Here's how the part is built. I have some questions about the finished solid (model axes, mm). Face numbers are marked on the shaded views. A direction names the side the tool comes from. Coordinates: 2 decimals unless noted, no trailing zeros. Loops run counter-clockwise (first coordinate to the right, second up) from the corner with the lowest first, then second, coordinate; pieces in that order, holes last.
Autodesk Fusion 360 part; units mm, degrees
sketch "Sketch1" plane through (0, 0, 0) normal (0, 0, 1) x (1, 0, 0)
  circle A0 centre (0, 0) radius 50
  circle A1 centre (0, 0) radius 67.5
  line L0 (-188.7298, 10) -> (-172.9129, 10)
  line L1 (-188.7147, -10.0585) -> (-172.8873, -10.0585)
  arc A2 (-172.8873, -10.0585) -> (-172.9129, 10) centre (-150, 0) ccw
  line L2 (190, -0.0314) -> (190, 0.0314)
  line L3 (188.7379, 9.9686) -> (172.9266, 9.9686)
  line L4 (188.7216, -10.0319) -> (172.8989, -10.0319)
  arc A3 (190, -0.0314) -> (190, 0.0314) centre (150, 0) ccw
  arc A4 (172.9266, 9.9686) -> (172.8989, -10.0319) centre (150, 0) ccw
  spline S0 degree 5 poles (-140.0807, 38.7506) (-138.5307, 38.3538) (-135.4703, 37.4053) (-128.0478, 36.7264) (-108.2202, 39.6197) (-74.7434, 48.8035) (-51.6098, 57.8401) (-40.0528, 63.8063) (-33.7446, 67.0737) (-30.5053, 68.5159) knots 0 0 0 0 0 0 0.2 0.4 0.6 0.8 1 1 1 1 1 1
  line L5 (-43.0547, 62.9285) -> (-17.9559, 74.1033)
  spline S1 degree 5 poles (-140.0807, -38.7506) (-138.5307, -38.3538) (-135.4703, -37.4053) (-127.9422, -36.808) (-107.6532, -40.0429) (-73.5767, -49.609) (-50.5343, -58.4957) (-39.5693, -64.0411) (-33.8156, -67.0222) (-30.867, -68.3537) knots 0 0 0 0 0 0 0.2 0.4 0.6 0.8 1 1 1 1 1 1
  line L6 (-42.1759, -63.2468) -> (-19.558, -73.4606)
  arc A5 (-188.7147, -10.0585) -> (-140.0807, -38.7506) centre (-150, 0) ccw
  arc A6 (-140.0807, 38.7506) -> (-188.7298, 10) centre (-150, 0) ccw
  spline S2 degree 5 poles (140.0807, 38.7506) (138.5307, 38.3538) (135.4703, 37.4053) (128.0873, 36.6912) (108.4368, 39.4331) (75.2221, 48.4229) (52.131, 57.4751) (40.4396, 63.5816) (33.9896, 66.9545) (30.6746, 68.4403) knots 0 0 0 0 0 0 0.2 0.4 0.6 0.8 1 1 1 1 1 1
  line L7 (43.2705, 62.7948) -> (18.0787, 74.0857)
  spline S3 degree 5 poles (140.0807, -38.7506) (138.5307, -38.3538) (135.4703, -37.4053) (128.1469, -36.639) (108.7618, -39.1583) (75.9243, -47.8755) (52.8578, -56.976) (40.9168, -63.3105) (34.2161, -66.8472) (30.768, -68.3983) knots 0 0 0 0 0 0 0.2 0.4 0.6 0.8 1 1 1 1 1 1
  line L8 (43.6214, -62.6164) -> (17.9147, -74.1802)
  arc A7 (188.7379, 9.9686) -> (140.0807, 38.7506) centre (150, 0) ccw
  arc A8 (140.0807, -38.7506) -> (188.7216, -10.0319) centre (150, 0) ccw
  arc A9 (-31.0302, -68.2798) -> (30.9809, -68.3022) centre (0, 0) ccw
  arc A10 (30.8878, 68.3443) -> (-30.6651, 68.4445) centre (0, 0) ccw
sketch "Esboço2" plane through (0, 0, 0) normal (0, 0, 1) x (1, 0, 0)
extrude "Extrusão1" add sketch "Sketch1" along normal blind 20 contours L0 L1 A2 L3 L4 A4 S0 L5 S1 L6 A5 A6 S2 L7 S3 L8 A7 A8 A9 A10
sketch "Esboço3" plane through (0, 0, 20) normal (0, 0, 1) x (1, 0, 0)
  circle A0 centre (0, 0) radius 67.5
  arc A1 (188.7379, 9.9686) -> (140.0807, 38.7506) centre (150, 0) ccw
  spline S0 degree 5 poles (140.0807, 38.7506) (138.5307, 38.3538) (135.4703, 37.4053) (128.0873, 36.6912) (108.4368, 39.4331) (75.3076, 48.3997) (52.2797, 57.4168) (40.5904, 63.503) (34.1559, 66.8675) (30.8878, 68.3443) knots 0 0 0 0 0 0 0.2 0.4 0.6 0.8 0.997426 0.997426 0.997426 0.997426 0.997426 0.997426
  arc A2 (30.8878, 68.3443) -> (-30.6651, 68.4445) centre (0, 0) ccw
  spline S1 degree 5 poles (-30.6651, 68.4445) (-33.8694, 67.009) (-40.1671, 63.7474) (-51.7241, 57.7955) (-74.8095, 48.7854) (-108.2202, 39.6197) (-128.0478, 36.7264) (-135.4703, 37.4053) (-138.5307, 38.3538) (-140.0807, 38.7506) knots -0.998025 -0.998025 -0.998025 -0.998025 -0.998025 -0.998025 -0.8 -0.6 -0.4 -0.2 0 0 0 0 0 0
  arc A3 (-140.0807, 38.7506) -> (-188.7298, 10) centre (-150, 0) ccw
  line L0 (-188.7298, 10) -> (-172.9129, 10)
  arc A4 (-172.8873, -10.0585) -> (-172.9129, 10) centre (-150, 0) ccw
  line L1 (-172.8873, -10.0585) -> (-188.7147, -10.0585)
  arc A5 (-188.7147, -10.0585) -> (-140.0807, -38.7506) centre (-150, 0) ccw
  spline S2 degree 5 poles (-140.0807, -38.7506) (-138.5307, -38.3538) (-135.4703, -37.4053) (-127.9422, -36.808) (-107.6532, -40.0429) (-73.6522, -49.5878) (-50.662, -58.4465) (-39.691, -63.9796) (-33.9434, -66.956) (-31.0302, -68.2798) knots 0 0 0 0 0 0 0.2 0.4 0.6 0.8 0.997784 0.997784 0.997784 0.997784 0.997784 0.997784
  arc A6 (-31.0302, -68.2798) -> (30.9809, -68.3022) centre (0, 0) ccw
  spline S3 degree 5 poles (30.9809, -68.3022) (34.382, -66.7597) (41.0646, -63.2323) (53.0003, -56.9198) (76.0055, -47.854) (108.7618, -39.1583) (128.1469, -36.639) (135.4703, -37.4053) (138.5307, -38.3538) (140.0807, -38.7506) knots -0.997529 -0.997529 -0.997529 -0.997529 -0.997529 -0.997529 -0.8 -0.6 -0.4 -0.2 0 0 0 0 0 0
  arc A7 (140.0807, -38.7506) -> (188.7216, -10.0319) centre (150, 0) ccw
  line L2 (188.7216, -10.0319) -> (172.8989, -10.0319)
  arc A8 (172.9266, 9.9686) -> (172.8989, -10.0319) centre (150, 0) ccw
  line L3 (172.9266, 9.9686) -> (188.7379, 9.9686)
  circle A9 centre (0, 0) radius 67.8
  circle A10 centre (0, 0) radius 50
  dimension "d17" = 135.6
  dimension "d18" = 100
extrude "Extrusão2" add sketch "Esboço3" against normal blind 10 contours A0
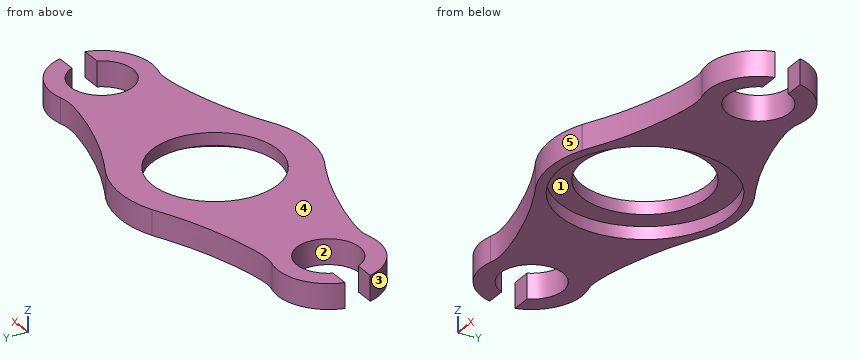
1. We'd pull the mould along X, two halves only. Please class the marked faces 3, 4 and 5: +X half, -X half, draft (parallel to the pull), parting line (faces both ways), or undercut.
2. I want a section at D-D (x = -4). Please give me the cut outline in (y, z).
3. I want a section at A-A (x = -150). Please give me the cut outline in (y, z), then the cut area to 3 significant figures.
4. I need wall thicknesses on line 1 along X through (y, z) = (-20.5, 7.25); line 2 along Y through (x, z) = (-150, 8.5); line 3 along X through (y, z) = (13, 18.5). Which ranges of each line are inside material? Lowest first, please.
5. On a 3-axis mill with a long thin cutter (end or side, diameter ignored), from which of +Z, -Z, +X, -X, +Y, -Y can I reach the whole of each face in a straight line? I mean the marked faces 1 and 2. Say none if no direction works.
6. I want a section at B-B (y = 0). Please give me the cut outline in (x, z).
7. For pin 1 (6 mm diameter, centred on y = -13, z = 4, fed in from +X); pin 2 (4 mm diameter, centred on x = 35.5, z = 6, fed in from -Y); pin 3 (1.5 mm diameter, centred on y = 6, z = 8.5, fed in from -X), each with a flat end and sliding along its axis, tell me the tip position at first contact or that it passes through.
Response values:
1. face 3: undercut
1. face 4: draft
1. face 5: parting line
2. outline: (-74.89, 0) - (-67.38, 0) - (-67.38, 10) - (-49.84, 10) - (-49.84, 20) - (-74.89, 20) - close; (49.84, 10) - (67.38, 10) - (67.38, 0) - (74.89, 0) - (74.89, 20) - (49.84, 20) - close
3. outline: (-40, 0) - (-25, 0) - (-25, 20) - (-40, 20) - close; (25, 0) - (40, 0) - (40, 20) - (25, 20) - close
3. area: 600 mm2
4. line 1: x = -184.35 to -164.31, -135.69 to -64.31, 64.31 to 135.69, 164.31 to 184.35
4. line 2: y = -40 to -25, 25 to 40
4. line 3: x = -187.83 to -171.35, -128.65 to -48.28, 48.28 to 128.65, 171.35 to 187.83
5. face 1: -Z
5. face 2: +Z, -Z
6. outline: (-125, 0) - (-67.5, 0) - (-67.5, 10) - (-50, 10) - (-50, 20) - (-125, 20) - close; (50, 10) - (67.5, 10) - (67.5, 0) - (125, 0) - (125, 20) - (50, 20) - close
7. pin 1: stops at x = 188.72
7. pin 2: stops at y = -67.11
7. pin 3: stops at x = -125.93
